Part print with two shaded views. Sizes in mm from the minimum x, y, z corner. A direction names the side the tool comes from. Coordinates: 2 decimals unless noted, no trailing zeros. Order: outer loops, then holes, each group sorted by start corner. A loop starts at its lowest first (then second) coordinate and runs counter-clockwise, first axis right, second up. Notation, with made-up numbers: (47.5, 2) - (58.5, 2) arc R14 ccw to (58.5, 26) - close; hole circle Ø2 at (10.25, 11). An arc over 180 degrees is marked (long way). One line per item, written item: value.
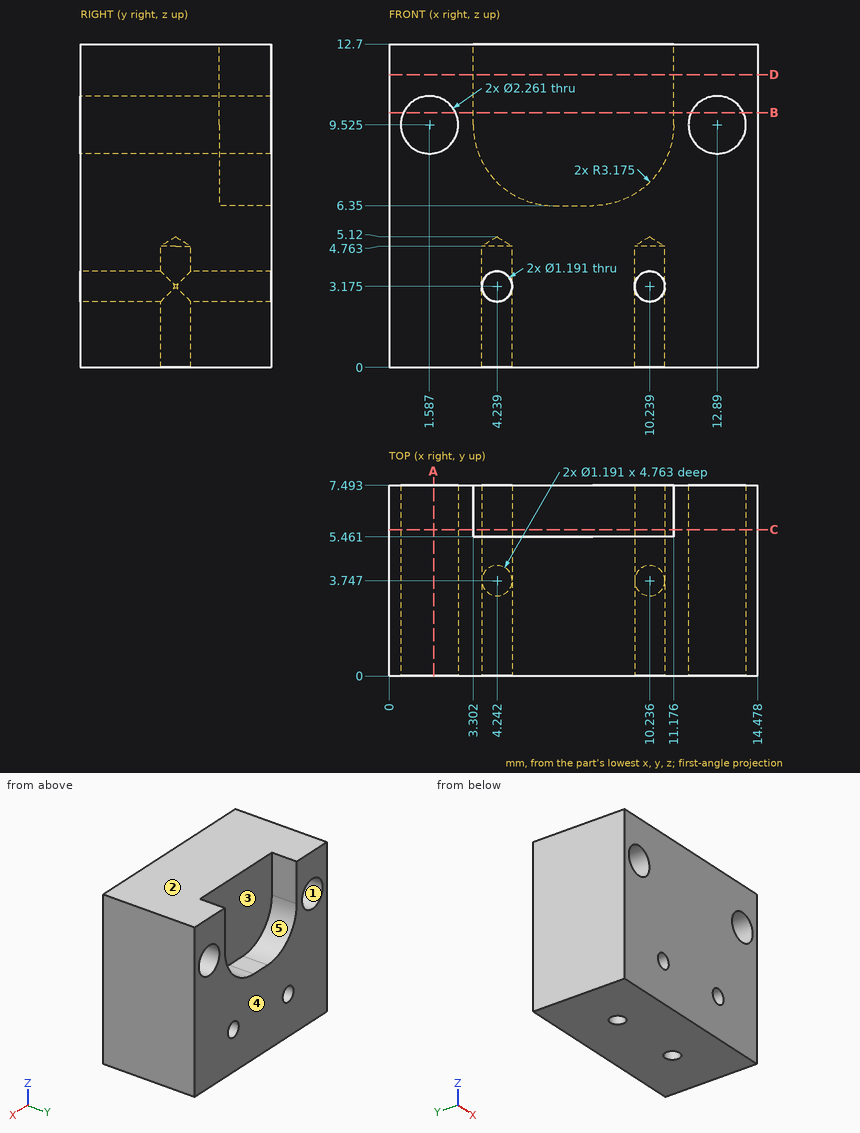
1. Flat gauge pins, fed straight in: P1, Ø1.9, axis at x = 6.5, z = 9, coming from the +Y side; P2, Ø1, axis at y = 5, z = 3.5, coming from the -X side; P3, Ø0.5, axis at x = 7.5, y = 6.5, coming from the +Z side. Where does each tip first touch, or does it go through?
Values found:
P1: stops at y = 5.46
P2: stops at x = 0
P3: stops at z = 6.35
2. Band-saw the part on D-D, the plane z = 11.5. Give the cut face in (x, y) (1 decimal).
Values found:
outline: (0, 0) - (14.5, 0) - (14.5, 7.5) - (11.2, 7.5) - (11.2, 5.5) - (3.3, 5.5) - (3.3, 7.5) - (0, 7.5) - close
3. 3-axis set-ups, long thin cutter, end or side, ignore diameter. For the marked faces 4 and 5: which of +Z, -Z, +X, -X, +Y, -Y reach the whole face in a straight line?
Values found:
face 4: +Z, -Z, +X, -X, +Y
face 5: +Z, +Y
4. Probe line 1 along X through (y, z) = (5, 9.5); line 2 along X through (y, z) = (2, 10.25) (1 decimal); line 3 along X through (y, z) = (7.25, 10.5) (1 decimal). List the from-to ranges inside material, lowest first.
Values found:
line 1: x = 0 to 0.46, 2.72 to 11.76, 14.02 to 14.48
line 2: x = 0 to 0.7, 2.5 to 12, 13.8 to 14.5
line 3: x = 0 to 1, 2.2 to 3.3, 11.2 to 12.3, 13.5 to 14.5
5. Band-saw the part on C-C, the plane y = 5.75. Count the separate pieces of the cut face and the enclosed holes in it, and give its area (3 significant figures).
Values found:
separate pieces: 1
enclosed holes: 4
area: 128 mm2
6. Two-plate mould, pull along Z, no slides. Class the marked faces 1, 2 and 3: pulls with the +Z half, pulls with the -Z half, needs draft (parallel to the pull), parting line crosses it, or undercut.
Values found:
face 1: undercut
face 2: pulls with the +Z half
face 3: needs draft
7. Band-saw the part on B-B, the plane z = 10. Give the cut face in (x, y) (1 decimal).
Values found:
outline: (0, 0) - (0.6, 0) - (0.6, 7.5) - (0, 7.5) - close; (2.6, 0) - (11.9, 0) - (11.9, 7.5) - (11.2, 7.5) - (11.2, 5.5) - (3.3, 5.5) - (3.3, 7.5) - (2.6, 7.5) - close; (13.9, 0) - (14.5, 0) - (14.5, 7.5) - (13.9, 7.5) - close
8. Band-saw the part on A-A, the plane x = 1.75. Give the cut face in (y, z).
Values found:
outline: (0, 0) - (7.49, 0) - (7.49, 8.41) - (0, 8.41) - close; (0, 10.64) - (7.49, 10.64) - (7.49, 12.7) - (0, 12.7) - close
